Build history of the part. All positions in model axes, mm. A direction names the side the tool comes from. Give positions to 0.01 mm unless a question says otherwise; leave off trailing zeros. Write each loop counter-clockwise with the first axis right and the second up, starting at its lowest first coordinate (ties: lowest second). Pieces come first, ordered by that corner, then holes. Notation, with made-up numbers: (-4.75, 3) -> (24.25, 3) arc R25 cw to (24.25, 27) -> close; hole circle Ø4 at (-11, 48). An arc over 180 degrees is marked (long way). Write item = value, one per line. Start each with the question number.
Q1. Saw through at B-B, the plane x = 24.5. List the corners of the cut face in (y, z) (3 decimals).
Q2. Tool access for faces 1 (the face through (74.191, 31, 38)), 2 (the face through (36.58, 23.6, 34.94)): list every direction of +Z, -Z, +X, -X, +Y, -Y with a clear straight run to the whole face (end or side of a thin tool).
Q3. Saw through at A-A, the plane y = 4. List the corners of the cut face in (x, z).
Q4. Wall check: line 1 (Z direction, x = 8, y = 25.5); line 2 (Y direction, x = 10, z = 39); line 3 (Z direction, x = 53, y = 23.5). Give the ranges that are in metal, low to high.
Q5. Drop flat-ended pins along their axis: P1, Ø8, axis at y = 25.91, z = 39.38, coming from the +X side; P2, Ø13.5, axis at y = 25.91, z = 39.38, coming from the +X side. Give the stop position or say it passes through.
Q6. Saw through at C-C, the plane y = 29.5. List the corners of the cut face in (x, z), then the cut area to 3 significant figures.
Q7. Mould opens along Y. For faces 3 (the face through (44, 51.734, 30)), 4 (the face through (89.191, 26, 27)), 5 (the face through (81.796, 33.066, 41.628)) say: pulls with the +Y half, pulls with the -Y half, needs draft (parallel to the pull), parting line crosses it, or undercut.
Q8. Saw through at D-D, the plane x = 77.5. List the corners of the cut face in (y, z) (3 decimals).
from build123d import *

# Parameters (mm, degrees)
F0_W           = 89.191195
F0_H           = 51.733698
F1_DEPTH       = 60
F2_R           = 5
F3_SIZE        = 5
F5_D           = 10
F5_CBORE_D     = 15
F5_CBORE_DEPTH = 15


with BuildPart() as f1:
    # F0 (on Top) → F1 (new body)
    with BuildSketch(Plane.XY):
        with Locations((44.595597, 25.866849)):
            Rectangle(F0_W, F0_H)
    extrude(amount=F1_DEPTH)

    # F2
    f2_edges = [f1.edges().sort_by_distance(p)[0] for p in [
        (89.191195, 25.866849, 60),
    ]]
    fillet(f2_edges, radius=F2_R)

    # F3
    f3_edges = [f1.edges().sort_by_distance(p)[0] for p in [
        (44.595597, 0, 0),
    ]]
    chamfer(f3_edges, length=F3_SIZE)

    # F5 (through all)
    with Locations(Plane.YZ.offset(89.191195)):
        with Locations((25.911886, 39.375003)):
            CounterBoreHole(F5_D / 2, F5_CBORE_D / 2, F5_CBORE_DEPTH)


solid = f1.part
Report:
q1.outline = (0, 5) -> (5, 0) -> (51.734, 0) -> (51.734, 60) -> (0, 60) -> close; hole circle Ø10 at (25.912, 39.375)
q2.face_1 = +X
q2.face_2 = +X, -X
q3.outline = (0, 1) -> (89.19, 1) -> (89.19, 55) arc R5 ccw to (84.19, 60) -> (0, 60) -> close
q4.line_1 = 0 to 34.39, 44.36 to 60
q4.line_2 = 0 to 20.93, 30.9 to 51.73
q4.line_3 = 0 to 35, 43.75 to 60
q5.P1 = through
q5.P2 = 74.19
q6.outline = (0, 0) -> (89.19, 0) -> (89.19, 32.79) -> (74.19, 32.79) -> (74.19, 35.89) -> (0, 35.89) -> close; (0, 42.86) -> (74.19, 42.86) -> (74.19, 45.96) -> (89.19, 45.96) -> (89.19, 55) arc R5 ccw to (84.19, 60) -> (0, 60) -> close
q6.area = 4,630 mm2
q7.face_3 = pulls with the +Y half
q7.face_4 = needs draft
q7.face_5 = undercut
q8.outline = (0, 5) -> (5, 0) -> (51.734, 0) -> (51.734, 60) -> (0, 60) -> close; hole circle Ø15 at (25.912, 39.375)
